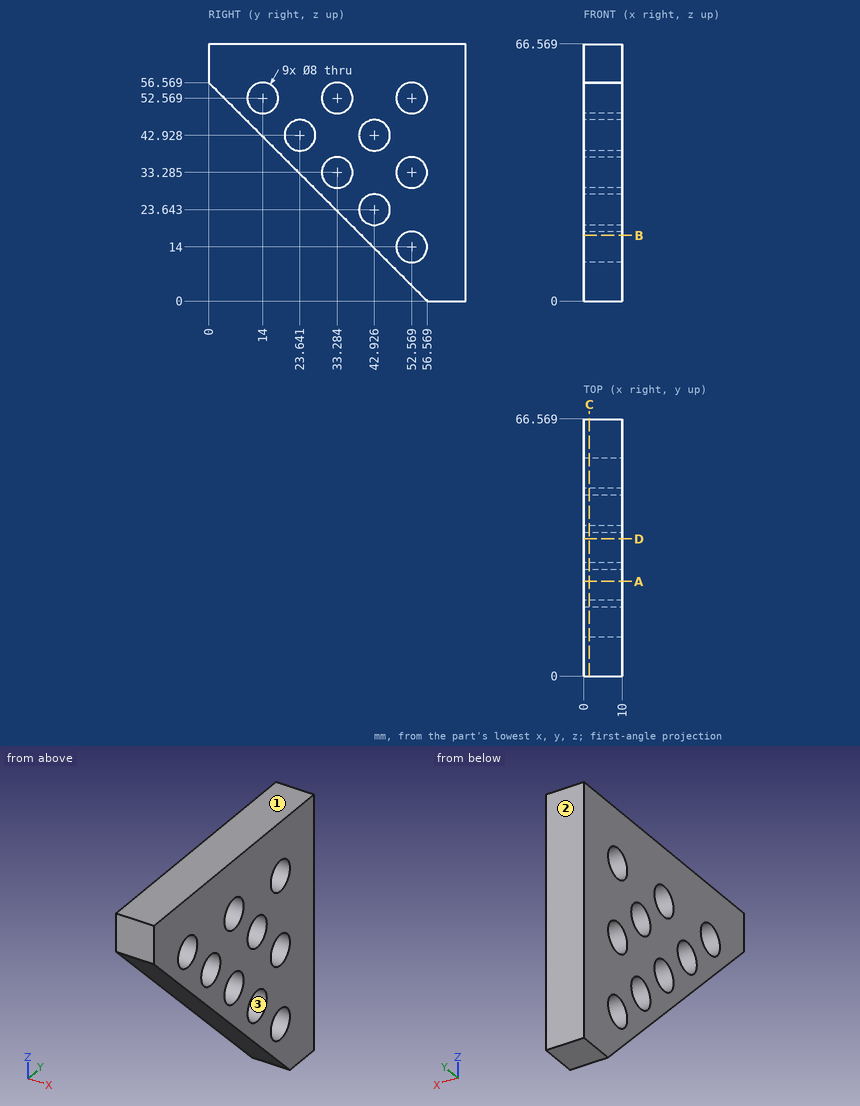
For this review, use the dimensioned drawing (mm, ordinates from the lowest corner) and the shaded views. Coordinates: 2 decimals unless noted, no trailing zeros. Loops run counter-clockwise (first coordinate to the right, second up) from the corner with the lowest first, then second, coordinate; pieces in that order, holes last. Notation, with made-up numbers: (-20, -30.5) - (-16, -30.5) arc R22 ccw to (-16, -13.5) - close; hole circle Ø7 at (34.25, -30). An arc over 180 degrees is marked (long way). Use CSV: the item, a comma, the result in double quotes. Start each with the question number.
1) Consider section A-A on y = 24.5. Write out the cut boundary in (x, z) (1 decimal).
2) Consider section D-D on y = 35.5. Write out the cut boundary in (x, z) (1 decimal), then the cut area to 3 significant figures.
3) For pin 1 Ø6.5 at (y, z) = (14, 52.57) entering from +X, flat-tipped, find the tip position at first contact; note if it passes through.
4) The part is to be moulded in two halves that separate along Y. For the marked faces 1, 2 and 3, say which applies: +Y half, -Y half, draft (parallel to the pull), parting line (faces both ways), or undercut.
5) Consider section C-C on x = 1.5. Give the number of separate pieces and of enclosed holes in the cut face, then the cut area to 3 significant figures.
6) Consider section B-B on z = 17. Write out the cut boundary in (x, y) (1 decimal), then the cut area to 3 significant figures.
7) Wall thickness on L1, parallel to Y at x = 8.5, z = 53.5 (1 decimal); L2, parallel to Y at x = 7.5, z = 49 (1 decimal); L3, parallel to Z at x = 2.25, y = 33 (1 decimal): over which ranges is each line inside the solid? List them lowest first. Write a range as from..to.
Geometry says:
1,outline,"(0, 32.1) - (10, 32.1) - (10, 39) - (0, 39) - close; (0, 46.8) - (10, 46.8) - (10, 66.6) - (0, 66.6) - close"
2,outline,"(0, 21.1) - (10, 21.1) - (10, 30) - (0, 30) - close; (0, 36.6) - (10, 36.6) - (10, 49.2) - (0, 49.2) - close; (0, 55.9) - (10, 55.9) - (10, 66.6) - (0, 66.6) - close"
2,area,"322 mm^2"
3,pin 1,"through"
4,face 1,"draft"
4,face 2,"+Y half"
4,face 3,"undercut"
5,separate pieces,"1"
5,enclosed holes,"9"
5,area,"2,380 mm^2"
6,outline,"(0, 39.6) - (10, 39.6) - (10, 49.9) - (0, 49.9) - close; (0, 55.2) - (10, 55.2) - (10, 66.6) - (0, 66.6) - close"
6,area,"217 mm^2"
7,L1,"3.1..10.1, 17.9..29.4, 37.2..48.7, 56.5..66.6"
7,L2,"7.6..12.2, 15.8..31.5, 35.1..50.8, 54.4..66.6"
7,L3,"23.6..29.3, 37.3..48.6, 56.6..66.6"
